Work out the finished part from the listing and answer in its coordinate system (mm). Round coordinates to 2 decimals unless told otherwise and drop trailing zeros. Write each loop counter-clockwise with the first axis right and the second up, starting at its lowest first coordinate (ties: lowest second). Pieces come first, ordered by that corner, then holes. Notation, with made-up numbers: M -16.5,71.25 L 24.5,71.25 A18 ccw 24.5,102.25 Z; hole C 6.25,12.25 d6. An arc over 180 degrees is marked long. Answer in a Markdown table with one row per item.
Autodesk Inventor part; units mm, degrees
ref_plane "YZ Plane" through (0, 0, 0) normal (1, 0, 0) x (0, 1, 0)
ref_plane "XZ Plane" through (0, 0, 0) normal (0, 1, 0) x (-1, 0, 0)
ref_plane "XY Plane" through (0, 0, 0) normal (0, 0, 1) x (1, 0, 0)
sketch "Sketch1" plane through (0, 0, 0) normal (0, 1, 0) x (-1, 0, 0)
  circle A0 centre (0, 0) radius 12 construction
  line L0 (0, 0) -> (0, -50) construction
  line L1 (-20, -16) -> (-34, -16) construction
  line L2 (-34, -16) -> (-34, -50) construction
  line L3 (-34, -50) -> (-20, -50) construction
  line L4 (-20, -50) -> (-20, -16) construction
  circle A1 centre (0, 0) radius 2
  arc A2 (5.2716, -2.8654) -> (-2.3397, 5.525) centre (0, 0) ccw
  line L5 (-34, -42) -> (-18.9731, -42)
  line L6 (5.2716, -2.8654) -> (-14.5801, -39.3878)
  line L7 (-2.3397, 5.525) -> (-35.9498, -8.7083)
  line L8 (-39, -13.3125) -> (-39, -37)
  arc A3 (-18.9731, -42) -> (-14.5801, -39.3878) centre (-18.9731, -37) ccw
  arc A4 (-39, -37) -> (-34, -42) centre (-34, -37) ccw
  arc A5 (-35.9498, -8.7083) -> (-39, -13.3125) centre (-34, -13.3125) ccw
  point P0 (-39, -42)
  point P1 (-16, -42)
  point P2 (-39, -10)
  dimension "d0" = 50
  dimension "d1" = 24
  dimension "d2" = 14
  dimension "d3" = 34
  dimension "d4" = 16
  dimension "d5" = 20
  dimension "d6" = 4
  dimension "d7" = 12
  dimension "d8" = 26
  dimension "d9" = 23
  dimension "d10" = 5
  dimension "d11" = 32
  dimension "d12" = 5
  dimension "d13" = 5
extrude "Extrusion1" add sketch "Sketch1" along normal blind 2
properties part number "flange_large"
1. The part is cut by section D-D (z = -23). Determine the outline of the cut face in (x, y).
Calculated:
| item | result |
|---|---|
| outline | M 5.67,0 L 39,0 L 39,2 L 5.67,2 Z |
2. Given pin 1 (5 mm diameter, centred on x = 2.5, z = -25, fed in from +Y); pin 2 (8 mm diameter, centred on x = 12.5, z = -27.5, fed in from -Y), each flat-ended and moving along its own axis, determine where each tip first touches the part or whether it passes through.
Calculated:
| item | result |
|---|---|
| pin 1 | passes through |
| pin 2 | stops at y = 0 |
3. The part is cut by section A-A (y = 1.3). Determine the outline of the cut face in (x, z) (1 decimal), plus the area to 3 significant figures.
Calculated:
| item | result |
|---|---|
| outline | M -5.3,-2.9 L 14.6,-39.4 A5 ccw 19,-42 L 34,-42 A5 ccw 39,-37 L 39,-13.3 A5 ccw 35.9,-8.7 L 2.3,5.5 A6 ccw Z; hole C 0,0 d4 |
| area | 1,380 mm² |
4. The part is cut by section C-C (x = 0). Determine the outline of the cut face in (y, z), plus the area to 3 significant figures.
Calculated:
| item | result |
|---|---|
| outline | M 0,-12.56 L 2,-12.56 L 2,-2 L 0,-2 Z; M 0,2 L 2,2 L 2,6 L 0,6 Z |
| area | 29.1 mm² |
5. Consider line 1 along Z through (x, y) = (0, 0.7); line 2 along Z through (x, y) = (18, 1.7); line 3 along X through (y, z) = (1.4, -26.5). Determine where each line is inside the solid, lowest interval first. Write a range as from..to.
Calculated:
| item | result |
|---|---|
| line 1 | z = -12.56..-2, 2..6 |
| line 2 | z = -41.9..-1.11 |
| line 3 | x = 7.57..39 |
6. Determine the mould class of faces 1 (the flat face through (4.515, 0.986, -20.871)), 2 (the flat face through (27, 1, -42)), 3 (the cylindrical face through (0, 1, 2)), 4 (the flat face through (18.909, 0.986, -1.492)) for opening direction X: released by +X, released by -X, zero draft, split by the parting line, or undercut.
Calculated:
| item | result |
|---|---|
| face 1 | released by -X |
| face 2 | zero draft |
| face 3 | undercut |
| face 4 | released by +X |
7. The part is cut by section B-B (z = -1). Determine the outline of the cut face in (x, y).
Calculated:
| item | result |
|---|---|
| outline | M -5.92,0 L -1.73,0 L -1.73,2 L -5.92,2 Z; M 1.73,0 L 17.75,0 L 17.75,2 L 1.73,2 Z |
